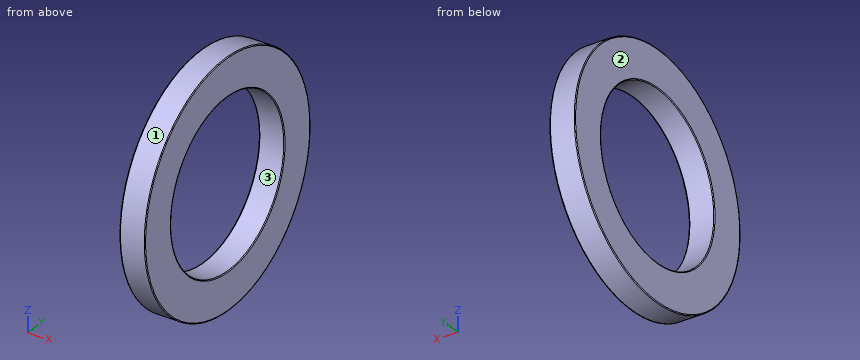
from build123d import *


with BuildPart() as part:
    # Croquis1 → Revolución1 (revolve)
    with BuildSketch(Plane(origin=(0, 0, 0), x_dir=(1, 0, 0), z_dir=(0, 1, 0)), mode=Mode.PRIVATE) as revoluci_n1_sk:
        with BuildLine():
            Line((0, 10.41), (1.505, 10.41))
            ThreePointArc((1.505, 10.41), (1.575710678, 10.439289322), (1.605, 10.51))
            Line((1.605, 10.51), (1.605, 15.05))
            ThreePointArc((1.605, 15.05), (1.575710678, 15.120710678), (1.505, 15.15))
            Line((1.505, 15.15), (-1.505, 15.15))
            ThreePointArc((-1.505, 15.15), (-1.575710678, 15.120710678), (-1.605, 15.05))
            Line((-1.605, 15.05), (-1.605, 10.51))
            ThreePointArc((-1.605, 10.51), (-1.575710678, 10.439289322), (-1.505, 10.41))
            Line((-1.505, 10.41), (0, 10.41))
        make_face()
    revolve(revoluci_n1_sk.sketch.rotate(Axis((0, 0, 0), (1, 0, 0)), 180), axis=Axis((0, 0, 0), (1, 0, 0)))


solid = part.part
Verification items for the finished model (mm, model axes). Face numbers are marked on the shaded views. Give positions to 0.01 mm unless a question says otherwise; leave off trailing zeros. Order: outer loops, then holes, each group sorted by start corner. A loop starts at its lowest first (then second) coordinate and runs counter-clockwise, first axis right, second up. Notation, with made-up numbers: (-11.75, 82.5) -> (8.25, 82.5) arc R31 cw to (8.25, 110.5) -> close; hole circle Ø6 at (50.25, 53). An arc over 180 degrees is marked (long way). Answer as CSV lines item,"result".
Q1. Sectioned sample at C-C on x = -0.55. Record the cut outline in (y, z), plus the area to 3 significant figures.
Solutions:
outline,"circle Ø30.3 at (0, 0); hole circle Ø20.82 at (0, 0)"
area,"381 mm²"
Q2. Release check for a two-part mould opening along Z. For the marked faces 1, 2 and 3 record: +Z half, -Z half, draft (parallel to the pull), parting line (faces both ways), or undercut.
Solutions:
face 1,"parting line"
face 2,"draft"
face 3,"undercut"
Q3. Depth check by flat-ended pin: pin 1 (1.5 mm diameter, centred on x = 0.5, z = 8, fed in from +Y); pin 2 (1 mm diameter, centred on x = -1, z = 11.5, fed in from -Y). Enter the tip coordinate at first touch or a pass-through.
Solutions:
pin 1,"stops at y = 13.3"
pin 2,"stops at y = -10.42"
Q4. Sectioned sample at A-A on y = 0. Record the cut outline in (x, z) (3 decimals), plus the area to 3 significant figures.
Solutions:
outline,"(-1.605, -15.05) arc R0.1 ccw to (-1.505, -15.15) -> (1.505, -15.15) arc R0.1 ccw to (1.605, -15.05) -> (1.605, -10.51) arc R0.1 ccw to (1.505, -10.41) -> (-1.505, -10.41) arc R0.1 ccw to (-1.605, -10.51) -> close; (-1.605, 10.51) arc R0.1 ccw to (-1.505, 10.41) -> (1.505, 10.41) arc R0.1 ccw to (1.605, 10.51) -> (1.605, 15.05) arc R0.1 ccw to (1.505, 15.15) -> (-1.505, 15.15) arc R0.1 ccw to (-1.605, 15.05) -> close"
area,"30.4 mm²"
Q5. Scan lines: probe 1 along Y at (x, z) = (0.35, 0); probe 2 along Y at (x, z) = (0.4, 11); probe 3 along Z at (x, y) = (-1.1, 8). Record each from-to range of solid material in increasing order.
Solutions:
probe 1,"y = -15.15 to -10.41, 10.41 to 15.15"
probe 2,"y = -10.42 to 10.42"
probe 3,"z = -12.87 to -6.66, 6.66 to 12.87"
